Read the model definition and answer for the solid it produces. Units are mm, in the model's axes. Round coordinates to 2 decimals unless told otherwise and drop trailing zeros. Write each loop counter-clockwise with the first axis right and the second up, starting at its lowest first coordinate (ties: lowest second). Pieces come first, ordered by that corner, then holes. Notation, with made-up numbers: (-20, -38.5) - (14, -38.5) arc R18 ccw to (14, -11.5) - close; hole circle Ø5 at (-3.5, 82.25). An arc over 180 degrees is marked (long way). Use one line per item in the form item = value. Start each with the question number.
1) The part is cut by section C-C, the plane y = -1.9. Give the vertices of the cut face in (x, z), plus the area to 3 significant figures.
2) Consider line 1 along Z through (x, y) = (49, -1.1); line 2 along Z through (x, y) = (-17.5, -1.55); line 3 along X through (y, z) = (-4.15, 38). Determine where each line is inside the solid, lowest interval first. Write a range as from..to.
3) The part is cut by section A-A, the plane z = 18. Give the vertices of the cut face in (x, y), plus the area to 3 significant figures.
4) The part is cut by section B-B, the plane x = 8. Give the vertices of the cut face in (y, z), plus the area to 3 significant figures.
5) The part is cut by section D-D, the plane x = -49. Give the vertices of the cut face in (y, z).
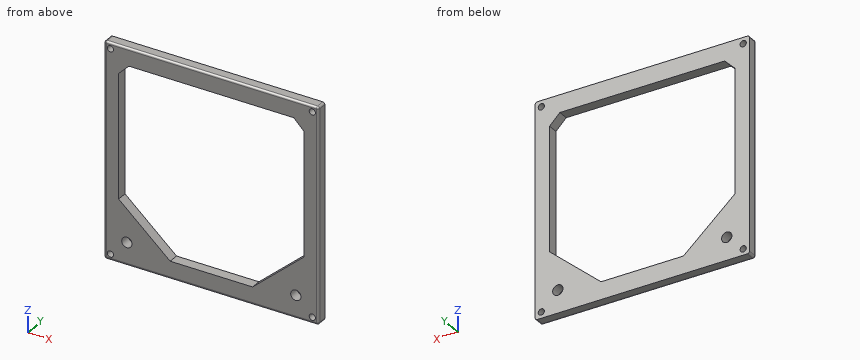
from build123d import *

# Parameters (mm, degrees)
F0_W        = 104
F0_H        = 104
F0_R        = 1.5
F0_R_2      = 2.5
F2_DEPTH    = 5
F2_FACE_W   = 104
F2_FACE_H   = 104
F2_FACE_R   = 1.5
F2_FACE_R_2 = 2.5
F3_DEPTH    = 25
F4_R        = 1


with BuildPart() as f2:
    # F0 (on Front) → F2 (new body)
    with BuildSketch(Plane.XZ):
        Rectangle(F0_W, F0_H)
        with Locations((-49, -49)):
            Circle(F0_R, mode=Mode.SUBTRACT)
        with Locations((-41, -41)):
            Circle(F0_R_2, mode=Mode.SUBTRACT)
        with Locations((49, -49)):
            Circle(F0_R, mode=Mode.SUBTRACT)
        with Locations((41, -41)):
            Circle(F0_R_2, mode=Mode.SUBTRACT)
        with Locations((-49, 49)):
            Circle(F0_R, mode=Mode.SUBTRACT)
        with Locations((49, 49)):
            Circle(F0_R, mode=Mode.SUBTRACT)
    extrude(amount=F2_DEPTH)

    # F1 (on Front) + F2_face (on face) → F3 (cut)
    with BuildSketch(Plane.XZ):
        Polygon((40, 43.5), (-40, 43.5), (-45, 38.5), (-45, -21.5), (-20, -43.5), (20, -43.5), (45, -21.5), (45, 38.5), align=None)
    with BuildSketch(Plane(origin=(0, -5, 0.149795), x_dir=(1, 0, 0), z_dir=(0, -1, 0))):
        with Locations((0, -0.149795)):
            Rectangle(F2_FACE_W, F2_FACE_H)
        with Locations((-49, -49.149795)):
            Circle(F2_FACE_R, mode=Mode.SUBTRACT)
        with Locations((-41, -41.149795)):
            Circle(F2_FACE_R_2, mode=Mode.SUBTRACT)
        with Locations((49, -49.149795)):
            Circle(F2_FACE_R, mode=Mode.SUBTRACT)
        with Locations((41, -41.149795)):
            Circle(F2_FACE_R_2, mode=Mode.SUBTRACT)
        with Locations((-49, 48.850205)):
            Circle(F2_FACE_R, mode=Mode.SUBTRACT)
        with Locations((49, 48.850205)):
            Circle(F2_FACE_R, mode=Mode.SUBTRACT)
    extrude(amount=F3_DEPTH, mode=Mode.SUBTRACT)

    # F4
    f4_edges = [f2.edges().sort_by_distance(p)[0] for p in [
        (-52, -2.5, 52),
        (-52, -5, 0),
        (0, -5, 52),
        (-52, -2.5, -52),
        (0, -5, -52),
        (52, -5, 0),
        (52, -2.5, 52),
        (52, -2.5, -52),
    ]]
    fillet(f4_edges, radius=F4_R)


solid = f2.part
Geometry results:
q1.outline = (-52, -51) arc R1 ccw to (-51, -52) - (51, -52) arc R1 ccw to (52, -51) - (52, 51) arc R1 ccw to (51, 52) - (-51, 52) arc R1 ccw to (-52, 51) - close; hole circle Ø3 at (-49, -49); hole circle Ø3 at (-49, 49); hole (-45, -21.5) - (-20, -43.5) - (20, -43.5) - (45, -21.5) - (45, 38.5) - (40, 43.5) - (-40, 43.5) - (-45, 38.5) - close; hole circle Ø5 at (-41, -41); hole circle Ø5 at (41, -41); hole circle Ø3 at (49, -49); hole circle Ø3 at (49, 49)
q1.area = 3,490 mm2
q2.line_1 = -52..-50.5, -47.5..47.5, 50.5..52
q2.line_2 = -52..-43.5, 43.5..52
q2.line_3 = -51.99..-45, 45..51.99
q3.outline = (-52, -4) arc R1 ccw to (-51, -5) - (-45, -5) - (-45, 0) - (-52, 0) - close; (45, -5) - (51, -5) arc R1 ccw to (52, -4) - (52, 0) - (45, 0) - close
q3.area = 69.6 mm2
q4.outline = (-5, -51) arc R1 ccw to (-4, -52) - (0, -52) - (0, -43.5) - (-5, -43.5) - close; (-5, 43.5) - (0, 43.5) - (0, 52) - (-4, 52) arc R1 ccw to (-5, 51) - close
q4.area = 84.6 mm2
q5.outline = (-5, -51) arc R1 ccw to (-4, -52) - (0, -52) - (0, -50.5) - (-5, -50.5) - close; (-5, -47.5) - (0, -47.5) - (0, 47.5) - (-5, 47.5) - close; (-5, 50.5) - (0, 50.5) - (0, 52) - (-4, 52) arc R1 ccw to (-5, 51) - close
